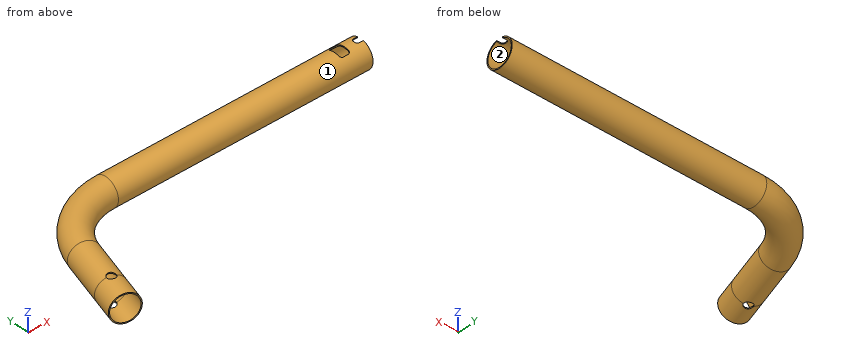
```python
from build123d import *

# Parameters (mm, degrees)
SKETCH3_R          = 11
SKETCH3_R_2        = 10.2
CUT_EXTRUDE1_REACH = 197.895
SKETCH4_R          = 3.3
SKETCH5_R          = 3.3
CUT_EXTRUDE2_DEPTH = 196.894862351


with BuildPart() as part:
    # Sweep2: sweep along a path in Sketch1
    with BuildLine(Plane.XY) as sweep2_path:
        Line((108.839588828, 0), (92.239588828, 0))
        Line((92.239588828, 0), (-92.239588828, 0))
        ThreePointArc((-92.239588828, 0), (-124.360019313, -10.591729527), (-143.88004565, -38.211927945))
        Line((-143.88004565, -38.211927945), (-154.760411172, -73.8))
        Line((-154.760411172, -73.8), (-160.324709574, -92))
    # Sketch3 → Sweep2 (sweep)
    with BuildSketch(Plane(origin=(92.239588828, 0, 0), x_dir=(0, 0, -1), z_dir=(1, 0, 0))):
        Circle(SKETCH3_R)
        Circle(SKETCH3_R_2, mode=Mode.SUBTRACT)
    sweep(path=sweep2_path.line)

    # Sketch4 → Cut-Extrude1 (cut, up to next)
    with BuildSketch(Plane.XY, mode=Mode.PRIVATE) as cut_extrude1_sk1:
        with Locations(Location((-154.760411172, -73.8, 0), (0, 0, 163))):
            Circle(SKETCH4_R)
    cut_extrude1_tool1 = extrude(cut_extrude1_sk1.sketch, amount=CUT_EXTRUDE1_REACH, mode=Mode.PRIVATE) & part.part
    # Sketch4 → Cut-Extrude1 (cut, up to next)
    with BuildSketch(Plane.XY, mode=Mode.PRIVATE) as cut_extrude1_sk2:
        with BuildLine():
            Line((108.839588828, 2.555545653), (108.839588828, -2.555545653))
            Line((108.839588828, -2.555545653), (105.639588828, -2.555545653))
            ThreePointArc((105.639588828, -2.555545653), (104.225375266, -1.969759216), (103.639588828, -0.555545653))
            Line((103.639588828, -0.555545653), (103.639588828, 0.555545653))
            ThreePointArc((103.639588828, 0.555545653), (104.225375266, 1.969759216), (105.639588828, 2.555545653))
            Line((105.639588828, 2.555545653), (108.839588828, 2.555545653))
        make_face()
    cut_extrude1_tool2 = extrude(cut_extrude1_sk2.sketch, amount=CUT_EXTRUDE1_REACH, mode=Mode.PRIVATE) & part.part
    # Sketch4 → Cut-Extrude1 (cut, up to next)
    with BuildSketch(Plane.XY, mode=Mode.PRIVATE) as cut_extrude1_sk3:
        with BuildLine():
            Line((90.239588828, -5.5), (94.239588828, -5.5))
            ThreePointArc((94.239588828, -5.5), (95.653802391, -4.914213562), (96.239588828, -3.5))
            Line((96.239588828, -3.5), (96.239588828, 3.5))
            ThreePointArc((96.239588828, 3.5), (95.653802391, 4.914213562), (94.239588828, 5.5))
            Line((94.239588828, 5.5), (90.239588828, 5.5))
            ThreePointArc((90.239588828, 5.5), (88.825375266, 4.914213562), (88.239588828, 3.5))
            Line((88.239588828, 3.5), (88.239588828, -3.5))
            ThreePointArc((88.239588828, -3.5), (88.825375266, -4.914213562), (90.239588828, -5.5))
        make_face()
    cut_extrude1_tool3 = extrude(cut_extrude1_sk3.sketch, amount=CUT_EXTRUDE1_REACH, mode=Mode.PRIVATE) & part.part
    add(cut_extrude1_tool1.solids().sort_by_distance((-154.760411, -73.8, 0))[0], mode=Mode.SUBTRACT)
    add(cut_extrude1_tool2.solids().sort_by_distance((106.388287, 0, 0))[0], mode=Mode.SUBTRACT)
    add(cut_extrude1_tool3.solids().sort_by_distance((92.239589, 0, 0))[0], mode=Mode.SUBTRACT)

    # Sketch5 → Cut-Extrude2 (cut, through all)
    with BuildSketch(Plane.XY):
        with Locations(Location((-154.760411172, -73.8, 0), (0, 0, 163))):
            Circle(SKETCH5_R)
    extrude(amount=-CUT_EXTRUDE2_DEPTH, mode=Mode.SUBTRACT)


solid = part.part
```
Source: CAD feature listing. Evaluate the final solid. Frame: model axes, mm. Face numbers are marked on the shaded views. Round coordinates to 2 decimals unless told otherwise and drop trailing zeros. Loops run counter-clockwise (first coordinate to the right, second up) from the corner with the lowest first, then second, coordinate; pieces in that order, holes last.
1. Mould query, pull axis Z, two halves, no side actions, for the marked faces 1 and 2. Classes: released by +Z, released by -Z, zero draft, split by the parting line, or undercut.
2. Section query B-B on x = 11. Output: boundary loops of the cut face in (y, z).
3. Contact query for flat-ended pins moving along their axis: pin 1 (5 mm diameter, centred on y = -53.5, z = 2.5, fed in from +X); pin 2 (0.5 mm diameter, centred on x = 92.5, z = 9, fed in from +Y); pin 3 (0.7 mm diameter, centred on y = 1, z = 10, fed in from +X). Output: stop coordinate, or through.
4. Ray query, L1, parallel to Y at x = -31.5, z = 0; L2, parallel to Z at x = 27, y = 3; L3, parallel to X at y = -47, z = -8. Return the intervals inside material, ascending.
5. Section query A-A on z = -3.5. Output: boundary loops of the cut face in (x, y), and give its area (3 significant figures).
Answers below:
1. face 1: split by the parting line
1. face 2: undercut
2. outline: circle Ø22 at (0, 0); hole circle Ø20.4 at (0, 0)
3. pin 1: stops at x = -136.46
3. pin 2: stops at y = 6.67
3. pin 3: stops at x = 103.8
4. L1: y = -11 to -10.2, 10.2 to 11
4. L2: z = -10.58 to -9.75, 9.75 to 10.58
4. L3: x = -154.46 to -153.18, -139.95 to -138.67
5. outline: (-170.3, -88.95) - (-169.49, -89.2) - (-153.04, -35.41) arc R63.58 cw to (-92.24, 9.58) - (108.84, 9.58) - (108.84, 10.43) - (-92.24, 10.43) arc R64.43 ccw to (-153.85, -35.16) - close; (-151.16, -94.8) - (-150.35, -95.05) - (-133.91, -41.26) arc R43.57 cw to (-92.24, -10.43) - (108.84, -10.43) - (108.84, -9.58) - (-92.24, -9.58) arc R44.42 ccw to (-134.72, -41.01) - close
5. area: 553 mm2
